```python
from build123d import *

# Parameters (mm, degrees)
F0_W           = 150
F0_H           = 150
F0_R           = 6.5
F0_R_2         = 14.75
F1_DEPTH       = 6
F2_R           = 9
F4_D           = 13
F4_CBORE_D     = 20
F4_CBORE_DEPTH = 3.5
F5_R           = 1
F6_R           = 0.5


with BuildPart() as f1:
    # F0 (on Top) → F1 (new body)
    with BuildSketch(Plane.XY):
        Rectangle(F0_W, F0_H)
        with Locations((-57, -57)):
            Circle(F0_R, mode=Mode.SUBTRACT)
        with Locations((57, -57)):
            Circle(F0_R, mode=Mode.SUBTRACT)
        with Locations((-57, 57)):
            Circle(F0_R, mode=Mode.SUBTRACT)
        Circle(F0_R_2, mode=Mode.SUBTRACT)
        with Locations((57, 57)):
            Circle(F0_R, mode=Mode.SUBTRACT)
    extrude(amount=F1_DEPTH)

    # F2
    f2_edges = [f1.edges().sort_by_distance(p)[0] for p in [
        (-75, -75, 3),
        (-75, 75, 3),
        (75, -75, 3),
        (75, 75, 3),
    ]]
    fillet(f2_edges, radius=F2_R)

    # F4 (through all)
    with Locations(Plane.XY.offset(6)):
        with Locations((-27.5, 27.5), (27.5, 27.5), (27.5, -27.5), (-27.5, -27.5)):
            CounterBoreHole(F4_D / 2, F4_CBORE_D / 2, F4_CBORE_DEPTH)

    # F5
    f5_edges = [f1.edges().sort_by_distance(p)[0] for p in [
        (-72.363961, 72.363961, 6),
        (0, 75, 6),
        (-75, 0, 6),
    ]]
    fillet(f5_edges, radius=F5_R)

    # F6
    f6_edges = [f1.edges().sort_by_distance(p)[0] for p in [
        (-75, 66, 2.5),
        (-75, 0, 5),
        (-75, 0, 0),
        (-75, -66, 2.5),
        (-66, -75, 2.5),
        (0, -75, 5),
        (0, -75, 0),
        (66, -75, 2.5),
    ]]
    fillet(f6_edges, radius=F6_R)


solid = f1.part
```
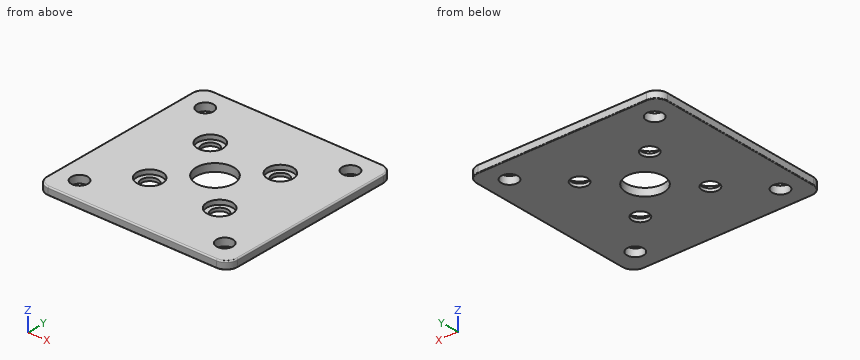
Geometry check sheet. Reference: the model listing, model coordinates, mm. Round coordinates to 2 decimals unless told otherwise and drop trailing zeros. Write each loop counter-clockwise with the first axis right and the second up, starting at its lowest first coordinate (ties: lowest second). Pieces come first, ordered by that corner, then holes. Notation, with made-up numbers: (67.25, 53.25) -> (90.25, 53.25) arc R23 cw to (90.25, 89.25) -> close; hole circle Ø8 at (-1, 31). An arc over 180 degrees is marked (long way). Put each result on its own line as item: value.
1) Thickness scan on probe 1 along Y at (x, z) = (-57, 2.65); probe 2 along Y at (x, z) = (-27.5, 4.55); probe 3 along X at (y, z) = (-22, 5.55). Record the ranges inside material, lowest first. Write a range as from..to.
Recorded:
probe 1: y = -75..-63.5, -50.5..50.5, 63.5..75
probe 2: y = -75..-37.5, -17.5..17.5, 37.5..75
probe 3: x = -74.84..-35.85, -19.15..19.15, 35.85..74.84
2) Cross-section at C-C, the plane z = 1.6. Give the number of separate pieces and of enclosed holes in the cut face, plus the area to 3 significant figures.
Recorded:
separate pieces: 1
enclosed holes: 9
area: 20,700 mm2
3) Depth check by flat-ended pin: P1, Ø16, axis at x = 24.5, y = 25, coming from the +Z side; P2, Ø11.5, axis at x = -27.5, y = 27.5, coming from the -Z side; P3, Ø6, axis at x = -23, y = -31, coming from the +Z side. Enter the tip coordinate at first touch or a pass-through.
Recorded:
P1: stops at z = 6
P2: passes through
P3: stops at z = 2.5
4) Cross-section at A-A, the plane y = 57. Enter the section's corners in (x, z).
Recorded:
outline: (-75, 0.5) arc R0.5 ccw to (-74.5, 0) -> (-63.5, 0) -> (-63.5, 6) -> (-74, 6) arc R1 ccw to (-75, 5) -> close; (-50.5, 0) -> (50.5, 0) -> (50.5, 6) -> (-50.5, 6) -> close; (63.5, 0) -> (74.5, 0) arc R0.5 ccw to (75, 0.5) -> (75, 5) arc R1 ccw to (74, 6) -> (63.5, 6) -> close
5) Cross-section at D-D, the plane y = 0. Enter the section's corners in (x, z).
Recorded:
outline: (-75, 0.5) arc R0.5 ccw to (-74.5, 0) -> (-14.75, 0) -> (-14.75, 6) -> (-74, 6) arc R1 ccw to (-75, 5) -> close; (14.75, 0) -> (74.5, 0) arc R0.5 ccw to (75, 0.5) -> (75, 5) arc R1 ccw to (74, 6) -> (14.75, 6) -> close
